```python
from build123d import *

# Parameters (mm, degrees)
SKETCH1_R           = 14.35
BOSS_EXTRUDE1_DEPTH = 100
CUT_EXTRUDE3_START  = -35
SKETCH2_R           = 13.97
CUT_EXTRUDE3_DEPTH  = 15


with BuildPart() as part:
    # Sketch1 → Boss-Extrude1 (new body)
    with BuildSketch(Plane(origin=(0, 0, 0), x_dir=(1, 0, 0), z_dir=(0, 1, 0))):
        with BuildLine():
            Line((16, -16), (-16, -16))
            Line((-16, -16), (-16, 0))
            ThreePointArc((-16, 0), (0, 16), (16, 0))
            Line((16, 0), (16, -16))
        make_face()
        with Locations(Location((0, 0, 0), (0, 0, 270))):
            Circle(SKETCH1_R, mode=Mode.SUBTRACT)
        Polygon((-13.566960835, -13.387527792), (-8.700031969, -13.387527792), (-13.566960835, -9.631173298), align=None, mode=Mode.SUBTRACT)
        Polygon((13.566960835, -13.387527792), (8.700031969, -13.387527792), (13.566960835, -9.631173298), align=None, mode=Mode.SUBTRACT)
    extrude(amount=BOSS_EXTRUDE1_DEPTH)

    # Sketch2 → Cut-Extrude3 (cut, symmetric)
    with BuildSketch(Plane.XY.offset(16).offset(CUT_EXTRUDE3_START)):
        with Locations((0, 54.866576619)):
            Circle(SKETCH2_R)
    extrude(amount=CUT_EXTRUDE3_DEPTH, both=True, mode=Mode.SUBTRACT)


solid = part.part
```
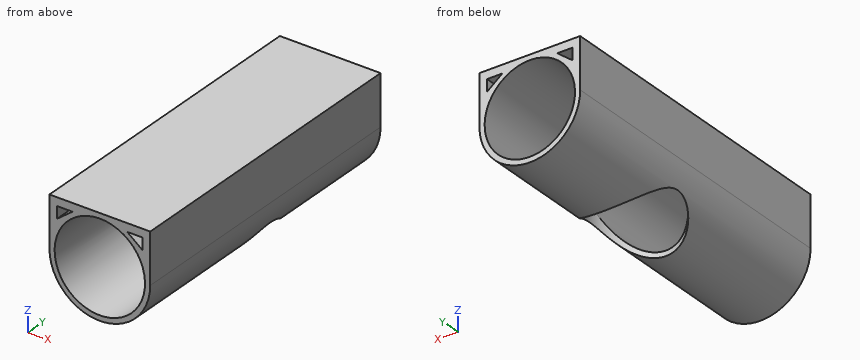
Could you check a few things on this model? Use its own coordinates, in mm. Round coordinates to 2 decimals unless told otherwise and drop trailing zeros. Loops run counter-clockwise (first coordinate to the right, second up) from the corner with the lowest first, then second, coordinate; pieces in that order, holes last. Notation, with made-up numbers: (66, -14.5) - (70, -14.5) arc R9 cw to (70, 1.5) - close; hole circle Ø11 at (1, 73.25). An arc over 180 degrees is marked (long way). Use CSV: the item, a comma, the result in double quotes.
Item 1: If we section it at A-A on x = 0: List the corners of the cut face in (y, z) for me.
Here are the results:
outline,"(0, -16) - (40.9, -16) - (40.9, -14.35) - (0, -14.35) - close; (0, 14.35) - (100, 14.35) - (100, 16) - (0, 16) - close; (68.84, -16) - (100, -16) - (100, -14.35) - (68.84, -14.35) - close"
Item 2: I need wall thicknesses on L1, parallel to X at y = 44, z = 4; L2, parallel to X at y = 75, z = 0. Which ranges of each line are inside material? Lowest first, please. Write a range as [from, to].
Here are the results:
L1,"x = [-16, -13.78], [13.78, 16]"
L2,"x = [-16, -14.35], [14.35, 16]"
Item 3: If we section it at D-D on z = 1: List the corners of the cut face in (x, y) for me.
Here are the results:
outline,"(-16, 0) - (-14.32, 0) - (-14.32, 100) - (-16, 100) - close; (14.32, 0) - (16, 0) - (16, 100) - (14.32, 100) - close"
Item 4: Will these pins go through, and if not, where does the flat tip stop? pin 1 (4 mm diameter, centred on x = 11.5, y = 27.5, fed in from -Z); pin 2 (5 mm diameter, centred on x = 10.5, y = 34, fed in from -Z); pin 3 (5 mm diameter, centred on y = 62, z = -7.5, fed in from +X).
Here are the results:
pin 1,"stops at z = -12.87"
pin 2,"stops at z = -13.86"
pin 3,"stops at x = 15.2"
Item 5: If we section it at C-C on z = -12: List the corners of the cut face in (x, y) for me, then the cut area to 3 significant figures.
Here are the results:
outline,"(-10.58, 0) - (-7.87, 0) - (-7.87, 43.32) arc R13.97 cw to (-10.58, 45.75) - close; (-10.58, 63.99) arc R13.97 cw to (-7.87, 66.41) - (-7.87, 100) - (-10.58, 100) - close; (7.87, 0) - (10.58, 0) - (10.58, 45.75) arc R13.97 cw to (7.87, 43.32) - close; (7.87, 66.41) arc R13.97 cw to (10.58, 63.99) - (10.58, 100) - (7.87, 100) - close"
area,"429 mm²"
Item 6: If we section it at B-B on y = 82.5: List the corners of the cut face in (x, z) for me.
Here are the results:
outline,"(-16, 0) arc R16 ccw to (16, 0) - (16, 16) - (-16, 16) - close; hole circle Ø28.7 at (0, 0); hole (-13.57, 9.63) - (-8.7, 13.39) - (-13.57, 13.39) - close; hole (8.7, 13.39) - (13.57, 9.63) - (13.57, 13.39) - close"
